Geometry: final body of the model. Coordinates: model frame, mm. Give positions to 0.01 mm unless a question says otherwise; leave off trailing zeros. Order: outer loops, then holes, each group sorted by start corner. A loop starts at its lowest first (then second) coordinate and runs counter-clockwise, first axis right, second up. Notation, with made-up numbers: (58, -8) - (108, -8) arc R24 cw to (108, 4) - close; hole circle Ø3 at (42, 59). An arc over 180 degrees is marked (long way). One line per question, with ' | ' between items. Start each with the question number.
from build123d import *

# Parameters (mm, degrees)
SKETCH2_R           = 50.8
BOSS_EXTRUDE1_DEPTH = 57.658
SKETCH3_R           = 5.08
CUT_EXTRUDE1_DEPTH  = 57.658
FILLET1_R           = 7.62


with BuildPart() as part:
    # Sketch2 → Boss-Extrude1 (new body)
    with BuildSketch(Plane(origin=(0, 0, 0), x_dir=(1, 0, 0), z_dir=(0, 1, 0))):
        with Locations(Location((0, 0, 0), (0, 0, 90))):
            Circle(SKETCH2_R)
    extrude(amount=BOSS_EXTRUDE1_DEPTH)

    # Sketch3 → Cut-Extrude1 (cut)
    with BuildSketch(Plane(origin=(0, 57.658, 0), x_dir=(1, 0, 0), z_dir=(0, 1, 0))):
        with Locations(Location((-41.011760438, 0.088591559, 0), (0, 0, 270))):
            Circle(SKETCH3_R)
    extrude(amount=-CUT_EXTRUDE1_DEPTH, mode=Mode.SUBTRACT)

    # Fillet1
    # the kernel refuses this fillet: 7.62 mm, written as the material it takes off along each edge
    with BuildSketch(Plane(origin=(-41.011760438, 57.658, -0.088591559), x_dir=(0, 0, 1), z_dir=(-1, 0, 0))) as fillet1_piece_1:
        with BuildLine():
            CenterArc((5.08 + FILLET1_R, -FILLET1_R), FILLET1_R, 90, 90)
            Line((5.08, -FILLET1_R), (5.08, 0))
            Line((5.08, 0), (5.08 + FILLET1_R, 0))
        make_face()
    revolve(axis=Axis((-41.011760438, 57.658, -0.088591559), (0, 1, 0)), mode=Mode.SUBTRACT)


solid = part.part
(1) Cut plane A-A, the plane y = 34. Return the cut outline in (x, z).
(2) Pull-direction query (Z, two-part tool) for faces 1 (the cylindrical face through (-35.975, 25.369, -0.75)), 2 (the flat face through (-1, 0, 1)), 3 (the cylindrical face through (30.911, 28.425, 40.313)); classes: +Z half, -Z half, draft (parallel to the pull), parting line (faces both ways), or undercut.
(3) Cut plane C-C, the plane z = 22. Return the cut outline in (x, y).
(4) Material intervals for line 1 along Z through (x, y) = (-1.5, 34.5); line 2 along Z through (x, y) = (26, 48.5); line 3 along X through (y, z) = (10.5, -6), sorted ascending. Write a range as from..to.
(5) Cut plane D-D, the plane y = 53.5. Return the cut outline in (x, z).
(6) Contact query for flat-ended pins moving along their axis: P1, Ø6, axis at y = 31.5, z = 23, coming from the -X side; P2, Ø1, axis at x = 14, y = 27.5, coming from the -Z side; P3, Ø12, axis at y = 18.5, z = -14, coming from the -X side; P4, Ø12, axis at x = -36.5, z = -29, coming from the -Y side. Output: stop coordinate, or through.
(7) Cut plane B-B, the plane x = -20.5. Return the cut outline in (y, z), plus the area to 3 significant figures.
Results are:
1) outline: circle Ø101.6 at (0, 0); hole circle Ø10.16 at (-41.01, -0.09)
2) face 1: undercut | face 2: draft | face 3: parting line
3) outline: (-45.79, 0) - (45.79, 0) - (45.79, 57.66) - (-45.79, 57.66) - close
4) line 1: -50.78..50.78 | line 2: -43.64..43.64 | line 3: -50.44..50.44
5) outline: circle Ø101.6 at (0, 0); hole circle Ø11.82 at (-41.01, -0.09)
6) P1: x = -46.7 | P2: z = -48.97 | P3: x = -50.17 | P4: y = 0
7) outline: (0, -46.48) - (57.66, -46.48) - (57.66, 46.48) - (0, 46.48) - close | area: 5,360 mm2
